Geometry check sheet. Reference: drawing and pictorial views, mm from the part's lowest x, y, z. A direction names the side the tool comes from. Coordinates: 2 decimals unless noted, no trailing zeros. Loops run counter-clockwise (first coordinate to the right, second up) from the corner with the lowest first, then second, coordinate; pieces in that order, holes last. Notation, with made-up numbers: (70.5, -17) -> (112.5, -17) arc R21 cw to (112.5, -13) -> close; hole circle Ø6 at (-18.75, 53.25). An arc over 180 degrees is marked (long way). Answer as a JSON object with one key per item and string values. Group by question number.
Q1. Cross-section at D-D on x = 7.5. Record the boundary of the cut face in (y, z).
Q2. Scan lines: L1, parallel to Z at x = 5.75, y = 20.5; L2, parallel to Y at x = 15.75, z = 40.5; L3, parallel to Y at x = 1.25, z = 4.5. Record each from-to range of solid material in increasing order.
Q3. Gauge pin test, flat ends, axial feed: pin 1 Ø1.5 at (x, y) = (19, 18) entering from +Z; pin 2 Ø3 at (y, z) = (13, 38.5) entering from +X; pin 3 Ø1.6 at (x, z) = (14, 40.5) entering from -Y. Record the tip position at first contact, or that the pin passes through.
Q4. Cross-section at C-C on z = 28. Record the boundary of the cut face in (x, y), and give its area (3 significant figures).
Q5. Cross-section at A-A on x = 13.5. Record the boundary of the cut face in (y, z), and give its area (3 significant figures).
Q6. Set-up check for the marked faces 1, 2, 3, 4 and 5: record each of +Z, -Z, +X, -X, +Y, -Y from which the full face is reachable in a straight line by a thin tool's end or side.
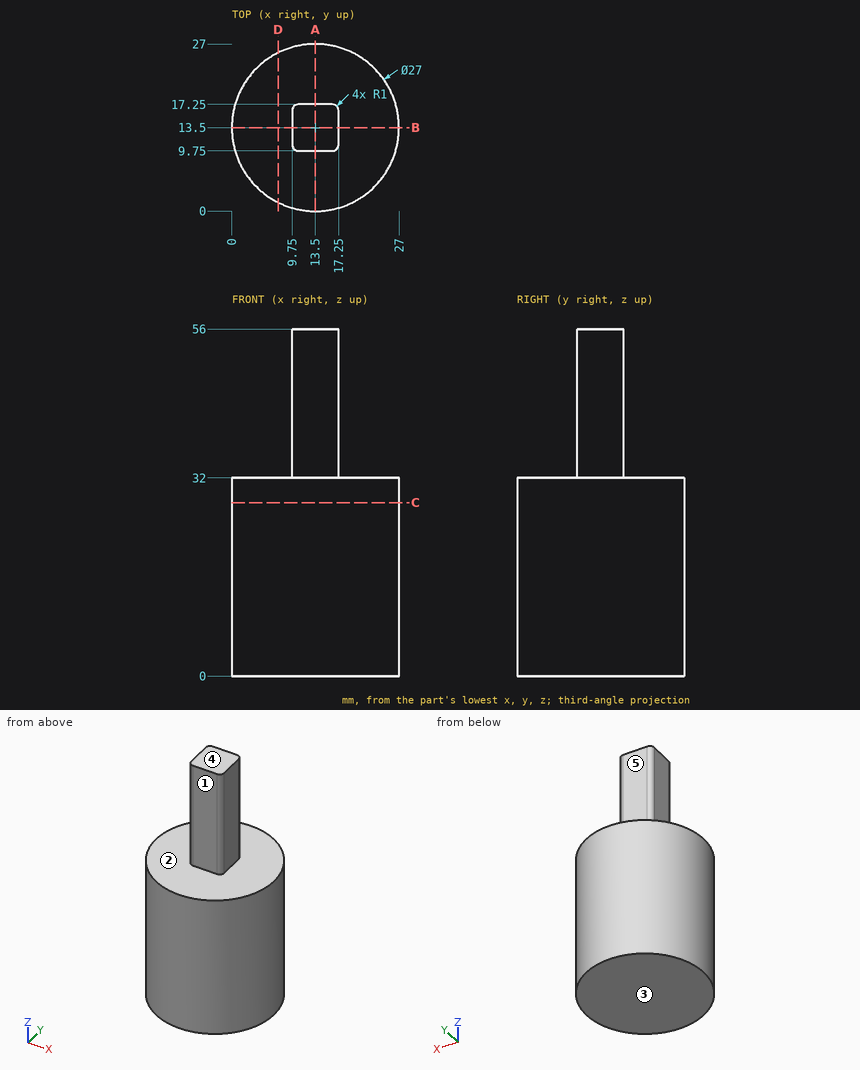
Computed values:
{
 "1": {"outline": "(1.41, 0) -> (25.59, 0) -> (25.59, 32) -> (1.41, 32) -> close"},
 "2": {"L1": "z = 0 to 32", "L2": "y = 9.75 to 17.25", "L3": "y = 7.83 to 19.17"},
 "3": {"pin 1": "stops at z = 32", "pin 2": "stops at x = 17.25", "pin 3": "stops at y = 9.75"},
 "4": {"outline": "circle Ø27 at (13.5, 13.5)", "area": "573 mm²"},
 "5": {"outline": "(0, 0) -> (27, 0) -> (27, 32) -> (17.25, 32) -> (17.25, 56) -> (9.75, 56) -> (9.75, 32) -> (0, 32) -> close", "area": "1,040 mm²"},
 "6": {"face 1": "+Z, +X, -X, -Y", "face 2": "+Z", "face 3": "-Z, +X, -X, +Y, -Y", "face 4": "+Z, +X, -X, +Y, -Y", "face 5": "+Z, +X, -X, +Y"}
}
